```python
from build123d import *

# Parameters (mm, degrees)
SKETCH1_R           = 2.41215
SKETCH1_R_2         = 2.6605
BOSS_EXTRUDE1_DEPTH = 8
BOSS_EXTRUDE2_DEPTH = 22.5
CUT_EXTRUDE1_DEPTH  = 22.5
SKETCH4_R           = 4.25
SKETCH4_R_2         = 2.6605
BOSS_EXTRUDE3_DEPTH = 4
CUT_EXTRUDE2_REACH  = 77.008
SKETCH6_R           = 10
BOSS_EXTRUDE4_DEPTH = 6
SKETCH7_R           = 2.6605
SKETCH7_W           = 16
SKETCH7_H           = 5
CUT_EXTRUDE3_DEPTH  = 76.00833287
SKETCH8_W           = 20.75
SKETCH8_H           = 22.5
CUT_EXTRUDE4_DEPTH  = 76.00833287
SKETCH9_W           = 26
SKETCH9_H           = 22.5
CUT_EXTRUDE5_DEPTH  = 2.25


with BuildPart() as part:
    # Sketch1 → Boss-Extrude1 (new body)
    with BuildSketch(Plane(origin=(0, 0, 0), x_dir=(1, 0, 0), z_dir=(0, 1, 0))):
        with BuildLine():
            Line((4, 0), (40, 0))
            ThreePointArc((40, 0), (42.828427125, 1.171572875), (44, 4))
            Line((44, 4), (44, 46))
            ThreePointArc((44, 46), (42.828427125, 48.828427125), (40, 50))
            Line((40, 50), (28, 50))
            ThreePointArc((28, 50), (25.171572875, 48.828427125), (24, 46))
            Line((24, 46), (24, 39))
            ThreePointArc((24, 39), (22.828427125, 36.171572875), (20, 35))
            Line((20, 35), (4, 35))
            ThreePointArc((4, 35), (1.171572875, 33.828427125), (0, 31))
            Line((0, 31), (0, 4))
            ThreePointArc((0, 4), (1.171572875, 1.171572875), (4, 0))
        make_face()
        with Locations(Location((34, 44, 0), (0, 0, 270))):
            Circle(SKETCH1_R, mode=Mode.SUBTRACT)
        with Locations(Location((14, 25.5, 0), (0, 0, 270))):
            Circle(SKETCH1_R_2, mode=Mode.SUBTRACT)
        with Locations(Location((10, 10, 0), (0, 0, 270))):
            Circle(SKETCH1_R, mode=Mode.SUBTRACT)
        with Locations(Location((22, 10, 0), (0, 0, 270))):
            Circle(SKETCH1_R, mode=Mode.SUBTRACT)
        with Locations(Location((39.63785, 10, 0), (0, 0, 270))):
            Circle(SKETCH1_R, mode=Mode.SUBTRACT)
    extrude(amount=BOSS_EXTRUDE1_DEPTH)

    # Sketch2 → Boss-Extrude2 (add)
    with BuildSketch(Plane(origin=(0, 8, 0), x_dir=(1, 0, 0), z_dir=(0, 1, 0))):
        with BuildLine():
            Line((4, 35), (20, 35))
            ThreePointArc((20, 35), (22.828427125, 36.171572875), (24, 39))
            Line((24, 39), (24, 46))
            ThreePointArc((24, 46), (25.171572838, 48.828427121), (27.999999942, 50))
            Line((27.999999942, 50), (40, 50))
            ThreePointArc((40, 50), (42.828427125, 48.828427125), (44, 46))
            Line((44, 46), (44, 4))
            ThreePointArc((44, 4), (42.828426987, 1.171572862), (39.999999786, 0))
            Line((39.999999786, 0), (4, 0))
            ThreePointArc((4, 0), (1.171572875, 1.171572875), (0, 4))
            Line((0, 4), (0, 31))
            ThreePointArc((0, 31), (1.171572875, 33.828427125), (4, 35))
        make_face()
        with BuildLine():
            Line((41.75, 46), (41.75, 4.000000214))
            ThreePointArc((41.75, 4.000000214), (41.237436804, 2.762563196), (39.999999786, 2.25))
            Line((39.999999786, 2.25), (4, 2.25))
            ThreePointArc((4, 2.25), (2.762563133, 2.762563133), (2.25, 4))
            Line((2.25, 4), (2.25, 31))
            ThreePointArc((2.25, 31), (2.762563133, 32.237436867), (4, 32.75))
            Line((4, 32.75), (20, 32.75))
            ThreePointArc((20, 32.75), (24.419417382, 34.580582618), (26.25, 39))
            Line((26.25, 39), (26.25, 46.000000058))
            ThreePointArc((26.25, 46.000000058), (26.762563116, 47.237436884), (27.999999942, 47.75))
            Line((27.999999942, 47.75), (40, 47.75))
            ThreePointArc((40, 47.75), (41.237436867, 47.237436867), (41.75, 46))
        make_face(mode=Mode.SUBTRACT)
    extrude(amount=BOSS_EXTRUDE2_DEPTH)

    # Sketch3 → Cut-Extrude1 (cut)
    with BuildSketch(Plane(origin=(0, 30.5, 0), x_dir=(1, 0, 0), z_dir=(0, 1, 0))):
        with BuildLine():
            Line((26.25, 50), (14, 50))
            Line((14, 50), (14, 36.5))
            ThreePointArc((14, 36.5), (6.221825407, 33.278174593), (3, 25.5))
            Line((3, 25.5), (0, 25.5))
            Line((0, 25.5), (0, 14.5))
            Line((0, 14.5), (14, 14.5))
            ThreePointArc((14, 14.5), (21.778174593, 17.721825407), (25, 25.5))
            Line((25, 25.5), (26.25, 25.5))
            Line((26.25, 25.5), (26.25, 50))
        make_face()
    extrude(amount=-CUT_EXTRUDE1_DEPTH, mode=Mode.SUBTRACT)

    # Sketch4 → Boss-Extrude3 (add)
    with BuildSketch(Plane(origin=(0, 30.5, 0), x_dir=(1, 0, 0), z_dir=(0, 1, 0))):
        with BuildLine():
            Line((28, 50), (40, 50))
            ThreePointArc((40, 50), (42.828427125, 48.828427125), (44, 46))
            Line((44, 46), (44, 4))
            ThreePointArc((44, 4), (42.828427125, 1.171572875), (40, 0))
            Line((40, 0), (4, 0))
            ThreePointArc((4, 0), (1.171572875, 1.171572875), (0, 4))
            Line((0, 4), (0, 31))
            ThreePointArc((0, 31), (1.171572875, 33.828427125), (4, 35))
            Line((4, 35), (20, 35))
            ThreePointArc((20, 35), (22.828427125, 36.171572875), (24, 39))
            Line((24, 39), (24, 46))
            ThreePointArc((24, 46), (25.171572875, 48.828427125), (28, 50))
        make_face()
        with Locations(Location((34, 44, 0), (0, 0, 61.927513064))):
            Circle(SKETCH4_R, mode=Mode.SUBTRACT)
        with Locations(Location((14, 25.5, 0), (0, 0, 270))):
            Circle(SKETCH4_R_2, mode=Mode.SUBTRACT)
        with Locations(Location((22, 10, 0), (0, 0, 270))):
            Circle(SKETCH4_R, mode=Mode.SUBTRACT)
        with Locations(Location((10, 10, 0), (0, 0, 270))):
            Circle(SKETCH4_R, mode=Mode.SUBTRACT)
        with Locations(Location((39.63785, 10, 0), (0, 0, 60.199834302))):
            Circle(SKETCH4_R, mode=Mode.SUBTRACT)
    extrude(amount=BOSS_EXTRUDE3_DEPTH)

    # Cut-Extrude2: up to this face of the body (flat: up to its plane)
    cut_extrude2_end = Plane(part.part.faces().sort_by_distance((23.387741141, 8, -22.067767212))[0])
    # Sketch5 → Cut-Extrude2 (cut, up to the picked face)
    with BuildSketch(Plane(origin=(0, 34.5, 0), x_dir=(1, 0, 0), z_dir=(0, 1, 0)), mode=Mode.PRIVATE) as cut_extrude2_sk1:
        with BuildLine():
            Line((39.63785, 14.25), (44, 14.25))
            Line((44, 14.25), (44, 5.75))
            Line((44, 5.75), (39.63785, 5.75))
            ThreePointArc((39.63785, 5.75), (35.38785, 10), (39.63785, 14.25))
        make_face()
    cut_extrude2_tool1 = split(extrude(cut_extrude2_sk1.sketch, amount=-CUT_EXTRUDE2_REACH, mode=Mode.PRIVATE), bisect_by=cut_extrude2_end, keep=Keep.BOTH, mode=Mode.PRIVATE)
    add(cut_extrude2_tool1.solids().sort_by(Axis((40.091525, 34.5, -10), (0, -1, 0)))[0], mode=Mode.SUBTRACT)

    # Sketch6 → Boss-Extrude4 (add)
    with BuildSketch(Plane(origin=(0, 8, 0), x_dir=(1, 0, 0), z_dir=(0, 1, 0))):
        with Locations(Location((14, 25.5, 0), (0, 0, 108.194872339))):
            Circle(SKETCH6_R)
    extrude(amount=BOSS_EXTRUDE4_DEPTH)

    # Sketch7 → Cut-Extrude3 (cut, through all)
    with BuildSketch(Plane.XZ):
        with Locations(Location((14, -25.5, 0), (0, 0, 90))):
            Circle(SKETCH7_R)
        with Locations((12, -37.5)):
            Rectangle(SKETCH7_W, SKETCH7_H)
    extrude(amount=-CUT_EXTRUDE3_DEPTH, mode=Mode.SUBTRACT)

    # Sketch8 → Cut-Extrude4 (cut, through all)
    with BuildSketch(Plane(origin=(44, 0, 0), x_dir=(0, 0, -1), z_dir=(1, 0, 0))):
        with Locations((24.625, 19.25)):
            Rectangle(SKETCH8_W, SKETCH8_H)
    extrude(amount=-CUT_EXTRUDE4_DEPTH, mode=Mode.SUBTRACT)

    # Sketch9 → Cut-Extrude5 (cut)
    with BuildSketch(Plane.XY):
        with Locations((22, 19.25)):
            Rectangle(SKETCH9_W, SKETCH9_H)
    extrude(amount=-CUT_EXTRUDE5_DEPTH, mode=Mode.SUBTRACT)


solid = part.part
```
Source: CAD feature listing. Evaluate the final solid. Frame: model axes, mm. A direction names the side the tool comes from. Round coordinates to 2 decimals unless told otherwise and drop trailing zeros. Write each loop counter-clockwise with the first axis right and the second up, starting at its lowest first coordinate (ties: lowest second). Pieces come first, ordered by that corner, then holes. Notation, with made-up numbers: M 65,32.25 L 102,32.25 A14 ccw 102,59.25 Z; hole C 85.25,39 d5. An arc over 180 degrees is marked long. Answer as a JSON object with one key per item and string values. Group by question number.
(1) Ray query, line 1 (X direction, y = 2, z = -10); line 2 (X direction, y = 31, z = -10); line 3 (Y direction, x = 13, z = -20). Return the intervals inside material, ascending. Write a range as [from, to].
(2) Mould query, pull axis Y, two halves, no side actions, for faces 1 (the cylindrical face through (22.797, 32.472, -36.141)), 2 (the flat face through (22, 0, -20)), 3 (the flat face through (34, 19, -47.75)). Classes: +Y half, -Y half, draft (parallel to the pull), parting line (faces both ways), or undercut.
(3) Section query A-A on z = -25.5. Output: boundary loops of the cut face in (x, y), then the cut area to 3 significant figures.
(4) Section query C-C on z = -18. Output: boundary loops of the cut face in (x, y).
(5) First-contact query: pin 1 (2.5 mm diameter, centred on y = 16.5, z = -0.5, fed in from +X); pin 2 (12 mm diameter, centred on y = 18.5, z = -40.5, fed in from -X); pin 3 (1.8 mm diameter, centred on x = 43, y = 19, fed in from +Z). Flat tips, straight axial feed; report the tip coordinate or a pass-through.
(6) Section query B-B on y = 5. Output: boundary loops of the cut face in (x, z), then the cut area to 3 significant figures.
(7) Section query D-D on y = 16. Output: boundary loops of the cut face in (x, z).
(8) Reachability of faces 4 (the flat face through (41.75, 19, -41)), 5 (the flat face through (26.25, 19, -48)), 6 (the flat face through (24, 32, -42)), 7 (the flat face through (2.25, 19, -9)) from +Z, -Z, +X, -X, +Y, -Y: full face, straight path, thin tool, end or side. Return the list, or none.
Computed values:
{
 "1": {"line 1": "[0, 7.59], [12.41, 19.59], [24.41, 37.23], [42.05, 44]", "line 2": "[0, 5.75], [14.25, 17.75], [26.25, 35.39]", "line 3": "[0, 8], [30.5, 34.5]"},
 "2": {"face 1": "draft", "face 2": "-Y half", "face 3": "undercut"},
 "3": {"outline": "M 0,0 L 11.34,0 L 11.34,8 L 0,8 Z; M 0,30.5 L 11.34,30.5 L 11.34,34.5 L 0,34.5 Z; M 16.66,0 L 44,0 L 44,8 L 16.66,8 Z; M 16.66,30.5 L 44,30.5 L 44,34.5 L 16.66,34.5 Z", "area": "464 mm^2"},
 "4": {"outline": "M 0,0 L 44,0 L 44,8 L 0,8 Z; M 0,30.5 L 44,30.5 L 44,34.5 L 0,34.5 Z"},
 "5": {"pin 1": "x = 43.31", "pin 2": "x = 26.25", "pin 3": "z = -0.6"},
 "6": {"outline": "M 0,-31 A4 ccw 4,-35 L 20,-35 A4 cw 24,-39 L 24,-46 A4 ccw 28,-50 L 40,-50 A4 ccw 44,-46 L 44,-4 A4 ccw 40,0 L 4,0 A4 ccw 0,-4 Z; hole C 10,-10 d4.82; hole C 14,-25.5 d5.32; hole C 22,-10 d4.82; hole C 34,-44 d4.82; hole C 39.64,-10 d4.82", "area": "1,730 mm^2"},
 "7": {"outline": "M 0,-14.25 L 2.25,-14.25 L 2.25,-4 A1.75 cw 4,-2.25 L 9,-2.25 L 9,0 L 4,0 A4 ccw 0,-4 Z; M 26.25,-49.6 A4 ccw 28,-50 L 40,-50 A4 ccw 44,-46 L 44,-35 L 41.75,-35 L 41.75,-46 A1.75 cw 40,-47.75 L 28,-47.75 A1.75 cw 26.25,-46 Z; M 35,-2.25 L 40,-2.25 A1.75 cw 41.75,-4 L 41.75,-5.75 L 44,-5.75 L 44,-4 A4 ccw 40,0 L 35,0 Z"},
 "8": {"face 4": "-X", "face 5": "+Z, -Z, -X", "face 6": "-Z, -X, +Y, -Y", "face 7": "-Z"}
}
